```python
from build123d import *

# Parameters (mm, degrees)
RESSALTO_EXTRUS_O1_DEPTH         = 35
FURO_DE_DI_METRO_11_0_11_1_D     = 11
FUROS_GUIA_COM_10_0MM1_D         = 10
FURO_DE_DI_METRO_11_0_11_2_D     = 11
FURO_DE_DI_METRO_11_0_11_2_DEPTH = 10
FURO_DE_DI_METRO_11_0_11_2_TIP   = 3.304733405
ESBO_O8_W                        = 0.2
ESBO_O8_H                        = 36.606458827
CORTE_EXTRUS_O1_DEPTH            = 0.2


with BuildPart() as part:
    # Esboço1 → Ressalto-extrusão1 (new body)
    with BuildSketch(Plane.XY):
        with BuildLine():
            Line((-199.997669575, -240.109131808), (-34.994179097, -240.27276126))
            ThreePointArc((-34.994179097, -240.27276126), (-0.031980607, -274.807449281), (34.998643265, -240.34217123))
            Line((34.998643265, -240.34217123), (200.002133743, -240.505800682))
            Line((200.002133743, -240.505800682), (199.972879413, -270.005786177))
            Line((199.972879413, -270.005786177), (57.635762375, -269.864634348))
            ThreePointArc((57.635762375, -269.864634348), (-0.061730772, -304.80743453), (-57.689806866, -269.750269132))
            Line((-57.689806866, -269.750269132), (-200.026923904, -269.609117302))
            Line((-200.026923904, -269.609117302), (-199.997669575, -240.109131808))
        make_face()
    extrude(amount=-RESSALTO_EXTRUS_O1_DEPTH)

    # Furo de diâmetro Ø11.0 (11)1 (through all)
    with Locations(Plane(origin=(-0.238306111, -240.30722771, 0), x_dir=(0.9999995082930158, -0.000991672187112085, 0), z_dir=(0.000991672187112085, 0.9999995082930158, 0))):
        with Locations((-179.759461687, 17.5), (-79.759461687, 17.5), (80.240538313, 17.5), (180.240538313, 17.5)):
            Hole(FURO_DE_DI_METRO_11_0_11_1_D / 2)

    # Furos-guia com Ø10.0mm1 (through all)
    with Locations(Plane(origin=(-0.267560441, -269.807213205, 0), x_dir=(-0.9999995082930158, 0.0009916721871120312, 0), z_dir=(-0.0009916721871120312, -0.9999995082930158, 0))):
        with Locations((129.759461687, 17.5), (-130.240538313, 17.5), (-221.181262437, -155.418379851)):
            Hole(FUROS_GUIA_COM_10_0MM1_D / 2)

    # Furo de diâmetro Ø11.0 (11)2
    with Locations(Plane(origin=(-0.267560441, -269.807213205, 0), x_dir=(-0.9999995082930158, 0.0009916721871120312, 0), z_dir=(-0.0009916721871120312, -0.9999995082930158, 0))):
        with Locations((129.759461687, 17.5), (-130.240538313, 17.5)):
            Hole(FURO_DE_DI_METRO_11_0_11_2_D / 2, depth=FURO_DE_DI_METRO_11_0_11_2_DEPTH)
            with Locations((0, 0, -(FURO_DE_DI_METRO_11_0_11_2_DEPTH + FURO_DE_DI_METRO_11_0_11_2_TIP / 2))):  # 118° drill point
                Cone(0, FURO_DE_DI_METRO_11_0_11_2_D / 2, FURO_DE_DI_METRO_11_0_11_2_TIP, mode=Mode.SUBTRACT)

    # Esboço8 → Corte-extrusão1 (cut)
    with BuildSketch(Plane(origin=(0, 0, -35), x_dir=(-1, 0, 0), z_dir=(0, 0, -1))):
        with Locations((-0.00272792, -289.800051975)):
            Rectangle(ESBO_O8_W, ESBO_O8_H)
    extrude(amount=-CORTE_EXTRUS_O1_DEPTH, mode=Mode.SUBTRACT)


solid = part.part
```
Work out the finished part from the listing and answer in its coordinate system (mm). Give positions to 0.01 mm unless a question says otherwise; leave off trailing zeros. Loops run counter-clockwise (first coordinate to the right, second up) from the corner with the lowest first, then second, coordinate; pieces in that order, holes last. Notation, with made-up numbers: (-13.75, -16) -> (-4.75, -16) arc R24 cw to (-4.75, 7) -> close; hole circle Ø9 at (10, 83.25). An arc over 180 degrees is marked (long way). Use CSV: the item, a comma, the result in double quotes.
1. The part is cut by section D-D (x = 14.5). Write down the section's boundary in (y, z).
Found:
outline,"(-303.17, -35) -> (-271.66, -35) -> (-271.66, 0) -> (-303.17, 0) -> close"
2. Flat-ended cylindrical pins translate along their axes: pin 1 Ø1.5 at (y, z) = (-266.5, -9) entering from -X; pin 2 Ø8 at (x, z) = (-112.5, -11) entering from +Y; pin 3 Ø4 at (x, z) = (-133, -12) entering from -Y. Find the tip coordinate at first contact, or state that the pin passes through.
Found:
pin 1,"x = -200.02"
pin 2,"y = -240.19"
pin 3,"y = -269.68"
3. The part is cut by section C-C (y = -246.5). State how many separate pieces and enclosed holes the cut face has, then the cut area to 3 significant figures.
Found:
separate pieces,"2"
enclosed holes,"6"
area,"11,100 mm^2"
4. Straight lines are drawn through the part: line 1 (Y direction, x = 179, z = -6); line 2 (X direction, y = -259, z = -29); line 3 (Y direction, x = 67.5, z = -22). For each, find the intervals that lie inside material, in ascending order.
Found:
line 1,"-269.98 to -240.48"
line 2,"-200.02 to -29.27, 29.27 to 199.98"
line 3,"-269.87 to -240.37"
5. The mould has two halves that part along Z. Classify faces 1 (the flat face through (3, -279, 0)), 2 (the cylindrical face through (-185.09, -255.08, -15.39)), 3 (the cylindrical face through (74.74, -255.34, -19.15)), 4 (the flat face through (-99, -265, -35)): +Z half, -Z half, draft (parallel to the pull), parting line (faces both ways), or undercut.
Found:
face 1,"+Z half"
face 2,"undercut"
face 3,"undercut"
face 4,"-Z half"
6. The part is cut by section A-A (z = -30). Write down the section's boundary in (x, y).
Found:
outline,"(-200.03, -269.61) -> (-57.69, -269.75) arc R65 ccw to (57.64, -269.86) -> (199.97, -270.01) -> (200, -240.51) -> (35, -240.34) arc R35 cw to (-34.99, -240.27) -> (-200, -240.11) -> close"
7. The part is cut by section B-B (y = -280.5). Write down the section's boundary in (x, z).
Found:
outline,"(-50.68, -35) -> (-0.1, -35) -> (-0.1, -34.8) -> (0.1, -34.8) -> (0.1, -35) -> (50.69, -35) -> (50.69, 0) -> (-50.68, 0) -> close"
